```python
from build123d import *

# Parameters (mm, degrees)
F0_W      = 53.5574629903
F0_H      = 30.0444331951
F1_DEPTH  = 25
F2_R      = 9.492451093
F3_DEPTH  = 17
F4_R      = 3
F5_R      = 7
F6_R      = 7
F7_R      = 7
F8_R      = 7
F11_W     = 10.4502402246
F11_H     = 5.4117300315
F12_DEPTH = 2


# Not quite as in the source:
# - the program builds the solid bodies; features that only make, move or delete a surface that nothing else refers to are left out


with BuildPart() as f1:
    # F0 (on Top) → F1 (new body)
    with BuildSketch(Plane.XY):
        with Locations((-33.1235192716, 21.5536148753)):
            Rectangle(F0_W, F0_H)
    extrude(amount=F1_DEPTH)

    # F2 (on face) → F3 (join)
    with BuildSketch(Plane.XY.offset(25)):
        with Locations((-17.996661365, 20.2366635203)):
            Circle(F2_R)
    extrude(amount=F3_DEPTH)

    # F4
    f4_edges = [f1.edges().sort_by_distance(p)[0] for p in [
        (-27.489112, 20.236664, 42),
    ]]
    fillet(f4_edges, radius=F4_R)

    # F5
    f5_edges = [f1.edges().sort_by_distance(p)[0] for p in [
        (-6.344788, 36.575831, 12.5),
    ]]
    fillet(f5_edges, radius=F5_R)

    # F6
    f6_edges = [f1.edges().sort_by_distance(p)[0] for p in [
        (-59.902251, 36.575831, 12.5),
    ]]
    fillet(f6_edges, radius=F6_R)

    # F7
    f7_edges = [f1.edges().sort_by_distance(p)[0] for p in [
        (-59.902251, 6.531398, 12.5),
    ]]
    fillet(f7_edges, radius=F7_R)

    # F8
    f8_edges = [f1.edges().sort_by_distance(p)[0] for p in [
        (-6.344788, 6.531398, 12.5),
    ]]
    fillet(f8_edges, radius=F8_R)

    # F11 (on face) → F12 (join)
    with BuildSketch(Plane(origin=(0, 36.5758314729, 0), x_dir=(-1, 0, 0), z_dir=(0, 1, 0))):
        with Locations((43.4804502875, 4.3853675597)):
            Rectangle(F11_W, F11_H)
    extrude(amount=F12_DEPTH)


solid = f1.part
```
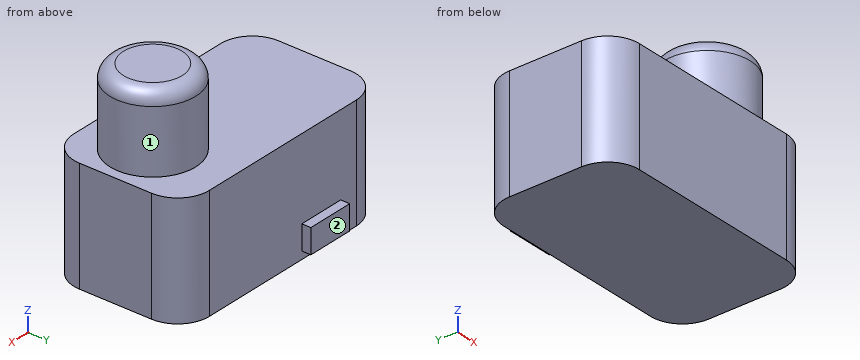
Check sheet for the modelled part. Datum: model origin and axes. Units: mm. Face numbers are marked on the shaded views. A direction names the side the tool comes from. Give positions to 0.01 mm unless a question says otherwise; leave off trailing zeros. Write each loop counter-clockwise with the first axis right and the second up, starting at its lowest first coordinate (ties: lowest second). Pieces come first, ordered by that corner, then holes. Notation, with made-up numbers: (73, -26) - (85, -26) arc R28 ccw to (85, 7) - close; hole circle Ø5 at (-8, 85.25). An arc over 180 degrees is marked (long way). Answer as a JSON object with one key per item and string values. Group by question number.
1) Thickness scan on probe 1 along Z at (x, y) = (-41, 30); probe 2 along Y at (x, z) = (-16, 4); probe 3 along X at (y, z) = (20, 36.5). Record the ranges inside material, lowest first. Write a range as from..to.
2) Sectioned sample at B-B (z = 4.5). Record the cut outline in (x, y), then the cut area to 3 significant figures.
3) Access from +Z, -Z, +X, -X, +Y, -Y to the whole of each face (thin tool, end or side, straight path). Record for the marked faces 1 and 2.
4) Sectioned sample at A-A (x = -45.5). Record the cut outline in (y, z).
5) Sectioned sample at D-D (y = 32). Record the cut outline in (x, z).
6) Depth check by flat-ended pin: P1, Ø5, axis at x = -23, y = 20.5, coming from the -Z side; P2, Ø0.6, axis at y = 37.5, z = 4, coming from the +X side; P3, Ø1.6, axis at x = -45.5, y = 38, coming from the +Z side; P4, Ø1, axis at x = -53, y = 16, coming from the +Z side. Enter the tip coordinate at first touch or a pass-through.
7) Sectioned sample at C-C (z = 10). Record the cut outline in (x, y), then the cut area to 3 significant figures.
Geometry results:
{
 "1": {"probe 1": "z = 0..25", "probe 2": "y = 6.53..36.58", "probe 3": "x = -27.49..-8.51"},
 "2": {"outline": "(-59.9, 13.53) arc R7 ccw to (-52.9, 6.53) - (-13.34, 6.53) arc R7 ccw to (-6.34, 13.53) - (-6.34, 29.58) arc R7 ccw to (-13.34, 36.58) - (-38.26, 36.58) - (-38.26, 38.58) - (-48.71, 38.58) - (-48.71, 36.58) - (-52.9, 36.58) arc R7 ccw to (-59.9, 29.58) - close", "area": "1,590 mm^2"},
 "3": {"face 1": "+Z", "face 2": "+Z, -Z, +X, -X, +Y"},
 "4": {"outline": "(6.53, 0) - (36.58, 0) - (36.58, 1.68) - (38.58, 1.68) - (38.58, 7.09) - (36.58, 7.09) - (36.58, 25) - (6.53, 25) - close"},
 "5": {"outline": "(-59.47, 0) - (-6.78, 0) - (-6.78, 25) - (-59.47, 25) - close"},
 "6": {"P1": "stops at z = 0", "P2": "stops at x = -38.26", "P3": "stops at z = 7.09", "P4": "stops at z = 25"},
 "7": {"outline": "(-59.9, 13.53) arc R7 ccw to (-52.9, 6.53) - (-13.34, 6.53) arc R7 ccw to (-6.34, 13.53) - (-6.34, 29.58) arc R7 ccw to (-13.34, 36.58) - (-52.9, 36.58) arc R7 ccw to (-59.9, 29.58) - close", "area": "1,570 mm^2"}
}
